```python
from build123d import *

# Parameters (mm, degrees)
F1_DEPTH = 360
F3_DEPTH = 30
F5_DEPTH = 30


with BuildPart() as f1:
    # F0 (on Front) → F1 (new body)
    with BuildSketch(Plane.XZ):
        Polygon((-30, 0), (0, 0), (0, 30), (-30, 38.602362), align=None)
    extrude(amount=F1_DEPTH)

    # F2 (on face) → F3 (cut)
    with BuildSketch(Plane(origin=(-30, 0, 0), x_dir=(0, -1, 0), z_dir=(-1, 0, 0))):
        Polygon((5.425208, 0), (0, 38.602362), (0, 0), align=None)
    extrude(amount=-F3_DEPTH, mode=Mode.SUBTRACT)

    # F4 (on face) → F5 (cut)
    with BuildSketch(Plane.XZ.offset(360)):
        Polygon((-20, 0), (-15, 0), (-10, 0), (-10, 32.867454), (-15, 34.301181), (-20, 35.734908), align=None)
    extrude(amount=-F5_DEPTH, mode=Mode.SUBTRACT)


solid = f1.part
```
Source: CAD feature listing. Evaluate the final solid. Frame: model axes, mm. A direction names the side the tool comes from. Coordinates: 2 decimals unless noted, no trailing zeros. Loops run counter-clockwise (first coordinate to the right, second up) from the corner with the lowest first, then second, coordinate; pieces in that order, holes last. Notation, with made-up numbers: M 14,22.25 L 53,22.25 A32 ccw 53,59.25 Z; hole C -32.5,-29 d7. An arc over 180 degrees is marked long. Use a Markdown table: item, result. Add a question column.
Q1. Section query A-A, the plane z = 21.5. Return loops of the section in (x, y), and give its area (3 significant figures).
Q2. Access query for faces 1 (the flat face through (-10, -345, 16)), 2 (the flat face through (-15.21, -2.75, 19.03)). Directions: +Z, -Z, +X, -X, +Y, -Y. A direction counts if a zero-diameter tool reaches every point of the face in a straight line with its end or side. Return the directions, or none.
Q3. Section query D-D, the plane z = 5.5. Return loops of the section in (x, y).
Q4. Section query C-C, the plane x = -5.75. Return loops of the section in (y, z).
Q5. Section query B-B, the plane y = -307.5. Return loops of the section in (x, z).
Q6. Draft query along X for faces 3 (the flat face through (-25, -360, 20)), 4 (the flat face through (-14.79, -177.48, 34.24)), 5 (the flat face through (-20, -345, 18)). Return one class per face: pulls with the +X half, pulls with the -X half, needs draft (parallel to the pull), parting line crosses it, or undercut.
Q7. Material intervals for L1, parallel to X at y = -343, z = 4.5; L2, parallel to Z at x = -19.75, y = -281; L3, parallel to Y at x = -28.25, z = 16.5, sorted ascending.
Q8. First-contact query: pin 1 (1 mm diameter, centred on x = -16, z = 23, fed in from +Y); pin 2 (4 mm diameter, centred on x = -4, y = -233, fed in from +Z); pin 3 (4 mm diameter, centred on x = -3, y = -224, fed in from +Z). Flat tips, straight axial feed; report the tip coordinate or a pass-through.
Result:
| question | item | result |
|---|---|---|
| 1 | outline | M -30,-360 L -20,-360 L -20,-330 L -10,-330 L -10,-360 L 0,-360 L 0,-2.4 L -30,-2.4 Z |
| 1 | area | 10,400 mm2 |
| 2 | face 1 | +Z, -Z, -Y |
| 2 | face 2 | -Z, +X, -X, +Y |
| 3 | outline | M -30,-360 L -20,-360 L -20,-330 L -10,-330 L -10,-360 L 0,-360 L 0,-4.65 L -30,-4.65 Z |
| 4 | outline | M -360,0 L -5.43,0 L -0.98,31.65 L -360,31.65 Z |
| 5 | outline | M -30,0 L 0,0 L 0,30 L -30,38.6 Z |
| 6 | face 3 | needs draft |
| 6 | face 4 | pulls with the +X half |
| 6 | face 5 | undercut |
| 7 | L1 | x = -30 to -20, -10 to 0 |
| 7 | L2 | z = 0 to 35.66 |
| 7 | L3 | y = -360 to -3.11 |
| 8 | pin 1 | stops at y = -2.12 |
| 8 | pin 2 | stops at z = 31.72 |
| 8 | pin 3 | stops at z = 31.43 |
